Geometry check sheet. Reference: the model listing, model coordinates, mm. A direction names the side the tool comes from. Give positions to 0.01 mm unless a question says otherwise; leave off trailing zeros. Loops run counter-clockwise (first coordinate to the right, second up) from the corner with the lowest first, then second, coordinate; pieces in that order, holes last. Notation, with made-up numbers: (-18.75, 78) -> (14.25, 78) arc R3 cw to (14.25, 82) -> close; hole circle Ø7 at (76.25, -2). An arc over 180 degrees is marked (long way). One line per question, with ' | ' between items.
from build123d import *

# Parameters (mm, degrees)
SKETCH_1_R          = 2.75
EXTRUDE_1_DEPTH     = 8
SKETCH_2_W          = 15.25
SKETCH_2_H          = 60
CUT_EXTRUDE_1_DEPTH = 10
FILLET_1_R          = 5
SKETCH_3_R          = 1.75
CUT_EXTRUDE_2_DEPTH = 123.800651464
SKETCH_4_R          = 5.525
CUT_EXTRUDE_3_DEPTH = 10


with BuildPart() as part:
    # 草图1 → 凸台-拉伸1 (new body)
    with BuildSketch(Plane.XY):
        Polygon((0, 0), (54, 0), (54, -52), (54, -110), (0, -110), align=None)
        with Locations((12, -106)):
            Circle(SKETCH_1_R, mode=Mode.SUBTRACT)
        with Locations((42, -106)):
            Circle(SKETCH_1_R, mode=Mode.SUBTRACT)
        with Locations((42, -76)):
            Circle(SKETCH_1_R, mode=Mode.SUBTRACT)
        with Locations((12, -76)):
            Circle(SKETCH_1_R, mode=Mode.SUBTRACT)
    extrude(amount=EXTRUDE_1_DEPTH)

    # 草图2 → 切除-拉伸1 (cut)
    with BuildSketch(Plane(origin=(0, 0, 0), x_dir=(-1, 0, 0), z_dir=(0, 0, -1))):
        with Locations((-7.625, -30)):
            Rectangle(SKETCH_2_W, SKETCH_2_H)
    extrude(amount=-CUT_EXTRUDE_1_DEPTH, mode=Mode.SUBTRACT)

    # 圆角1
    fillet_1_edges = [part.edges().sort_by_distance(p)[0] for p in [
        (15.25, 0, 4),
        (0, -60, 4),
        (15.25, -60, 4),
        (54, 0, 4),
    ]]
    fillet(fillet_1_edges, radius=FILLET_1_R)

    # 草图3 → 切除-拉伸2 (cut, through all)
    with BuildSketch(Plane(origin=(0, 0, 0), x_dir=(-1, 0, 0), z_dir=(0, 0, -1))):
        with Locations((-20, -4)):
            Circle(SKETCH_3_R)
        with Locations((-34, -4)):
            Circle(SKETCH_3_R)
        with Locations((-34, -56)):
            Circle(SKETCH_3_R)
        with Locations((-20, -56)):
            Circle(SKETCH_3_R)
    extrude(amount=-CUT_EXTRUDE_2_DEPTH, mode=Mode.SUBTRACT)

    # 草图4 → 切除-拉伸3 (cut)
    with BuildSketch(Plane(origin=(0, 0, 0), x_dir=(-1, 0, 0), z_dir=(0, 0, -1))):
        with Locations((-36.55, -30)):
            Circle(SKETCH_4_R)
    extrude(amount=-CUT_EXTRUDE_3_DEPTH, mode=Mode.SUBTRACT)


solid = part.part
Item 1: Sectioned sample at D-D (x = 12). Record the cut outline in (y, z), plus the area to 3 significant figures.
Result:
outline: (-110, 0) -> (-108.75, 0) -> (-108.75, 8) -> (-110, 8) -> close; (-103.25, 0) -> (-78.75, 0) -> (-78.75, 8) -> (-103.25, 8) -> close; (-73.25, 0) -> (-59.68, 0) -> (-59.68, 8) -> (-73.25, 8) -> close | area: 315 mm2
Item 2: Scan lines: probe 1 along X at (y, z) = (-75, 6); probe 2 along Y at (x, z) = (35.5, 1.5); probe 3 along Y at (x, z) = (34, 4.5). Record each from-to range of solid material in increasing order.
Result:
probe 1: 0 to 9.44, 14.56 to 39.44, 44.56 to 54 | probe 2: -110 to -56.9, -55.1 to -35.42, -24.58 to -4.9, -3.1 to 0 | probe 3: -110 to -57.75, -54.25 to -34.9, -25.1 to -5.75, -2.25 to 0
Item 3: Sectioned sample at A-A (y = -4). Record the cut outline in (x, z), plus the area to 3 significant figures.
Result:
outline: (15.35, 0) -> (18.25, 0) -> (18.25, 8) -> (15.35, 8) -> close; (21.75, 0) -> (32.25, 0) -> (32.25, 8) -> (21.75, 8) -> close; (35.75, 0) -> (53.9, 0) -> (53.9, 8) -> (35.75, 8) -> close | area: 252 mm2
Item 4: Depth check by flat-ended pin: pin 1 Ø2.5 at (y, z) = (-40.5, 5.5) entering from -X; pin 2 Ø2.5 at (x, z) = (6.5, 4) entering from +Y. Enter the tip coordinate at first touch or a pass-through.
Result:
pin 1: x = 15.25 | pin 2: y = -60
Item 5: Sectioned sample at B-B (x = 37). Record the cut outline in (y, z).
Result:
outline: (-110, 0) -> (-35.51, 0) -> (-35.51, 8) -> (-110, 8) -> close; (-24.49, 0) -> (0, 0) -> (0, 8) -> (-24.49, 8) -> close
Item 6: Set-up check for faces 1 (the face through (27, -54, 8)), 2 (the face through (15.25, -30, 4)): record each of +Z, -Z, +X, -X, +Y, -Y from which the full face is reachable in a straight line by a thin tool's end or side.
Result:
face 1: +Z, +X, -X, +Y, -Y | face 2: +Z, -Z, -X, +Y
Item 7: Sectioned sample at C-C (z = 6). Give the number of separate pieces and of enclosed holes in the cut face, plus the area to 3 significant figures.
Result:
separate pieces: 1 | enclosed holes: 9 | area: 4,780 mm2
Item 8: Release check for a two-part mould opening along Y. For faces 3 (the face through (11.642, -73.273, 3.944)), 4 (the face through (8, -60, 4)), 5 (the face through (27, -54, 0)) record: pulls with the +Y half, pulls with the -Y half, needs draft (parallel to the pull), parting line crosses it, or undercut.
Result:
face 3: undercut | face 4: pulls with the +Y half | face 5: needs draft
